Model file for the job. Use its own axes, mm. Round coordinates to 2 decimals unless told otherwise and drop trailing zeros. Write each loop counter-clockwise with the first axis right and the second up, starting at its lowest first coordinate (ties: lowest second). Pieces come first, ordered by that corner, then holes. Notation, with made-up numbers: (44, 32) - (51, 32) arc R4 cw to (51, 39) - close; hole circle Ø7 at (-7, 61). An arc over 180 degrees is marked (long way). Answer as a JSON object with one key per item and string values. Group by question number.
from build123d import *

# Parameters (mm, degrees)
SKETCH_1_R               = 22.5
SKETCH_1_R_2             = 19.5
EXTRUDE_1_DEPTH          = 120
SKETCH_3_R               = 1
CUT_EXTRUDE_1_DEPTH      = 10
PATTERN_CIRCULAR_1_COUNT = 4


with BuildPart() as part:
    # Эскиз1 → Бобышка-Вытянуть1 (new body)
    with BuildSketch(Plane(origin=(0, 0, 0), x_dir=(0, 0, -1), z_dir=(1, 0, 0))):
        Circle(SKETCH_1_R)
        Circle(SKETCH_1_R_2, mode=Mode.SUBTRACT)
    extrude(amount=EXTRUDE_1_DEPTH)

    # Эскиз3 → Вырез-Вытянуть1 (cut)
    with BuildSketch(Plane(origin=(0, 22.5, 0), x_dir=(1, 0, 0), z_dir=(0, 1, 0))):
        with Locations(Location((6, 0, 0), (0, 0, 270))):
            Circle(SKETCH_3_R)
        with Locations(Location((114, 0, 0), (0, 0, 270))):
            Circle(SKETCH_3_R)
    cut_extrude_1 = extrude(amount=-CUT_EXTRUDE_1_DEPTH, mode=Mode.SUBTRACT)

    # Круговой массив1: Вырез-Вытянуть1 ×4 about axis
    pattern_circular_1_axis = Axis((120, 0, 0), (-1, 0, 0))
    for i in range(1, PATTERN_CIRCULAR_1_COUNT):
        add(cut_extrude_1.rotate(pattern_circular_1_axis, i * 360 / PATTERN_CIRCULAR_1_COUNT), mode=Mode.SUBTRACT)


solid = part.part
(1) Slice it at C-C (x = 65). Write the cut outline in (y, z).
(2) Drill centre lines: line 1 (X direction, y = 0, z = -20.5); line 2 (Y direction, x = 27, z = -1); line 3 (Z direction, x = 114, y = 20.8). Where is each one in solid material? Low to high. Write a range as from..to.
(3) Flat gauge pins, fed straight in: pin 1 (3 mm diameter, centred on x = 114, y = 0, fed in from -Z); pin 2 (1 mm diameter, centred on x = 36.5, z = 17.5, fed in from +Y); pin 3 (1.5 mm diameter, centred on x = 19.5, z = -12.5, fed in from -Y); pin 4 (3 mm diameter, centred on x = 88.5, y = -17, fed in from -Z). Where does each tip first touch, or does it go through?
(4) Pull direction Y, two halves, no side cores. Call faces 1 (the cylindrical face through (59.16, 5.86, -18.6)), 2 (the flat face through (120, 10, 17)), 3 (the cylindrical face through (59.16, -19.961, -10.382)): pulls with the +Y half, pulls with the -Y half, needs draft (parallel to the pull), parting line crosses it, or undercut.
(5) Slice it at A-A (y = -3). Write the cut outline in (x, z).
(6) Slice it at B-B (z = 3.5). Write the cut outline in (x, y).
Answer:
{
 "1": {"outline": "circle Ø45 at (0, 0); hole circle Ø39 at (0, 0)"},
 "2": {"line 1": "0..5, 7..113, 115..120", "line 2": "-22.48..-19.47, 19.47..22.48", "line 3": "-8.58..-1, 1..8.58"},
 "3": {"pin 1": "z = -22.5", "pin 2": "y = 14.74", "pin 3": "y = -19.19", "pin 4": "z = -16.31"},
 "4": {"face 1": "undercut", "face 2": "needs draft", "face 3": "parting line crosses it"},
 "5": {"outline": "(0, -22.3) - (120, -22.3) - (120, -19.27) - (0, -19.27) - close; (0, 19.27) - (120, 19.27) - (120, 22.3) - (0, 22.3) - close"},
 "6": {"outline": "(0, -22.23) - (120, -22.23) - (120, -19.18) - (0, -19.18) - close; (0, 19.18) - (120, 19.18) - (120, 22.23) - (0, 22.23) - close"}
}
